Can you work these out from the model? Positions are in its coordinate system, mm. Face numbers are marked on the shaded views. A direction names the side the tool comes from. Coordinates: 2 decimals unless noted, no trailing zeros. Order: outer loops, then holes, each group sorted by start corner. A loop starts at its lowest first (then second) coordinate and runs counter-clockwise, first axis right, second up. Notation, with made-up numbers: M 69.25,-6.5 L 97.25,-6.5 A17 cw 97.25,17.5 Z; hole C 84,18.5 d11. An arc over 180 degrees is marked long. Answer as CSV lines item,"result". Start each with the question number.
1. I need wall thicknesses on line 1 along Y through (x, z) = (0, -16.3); line 2 along Y through (x, z) = (0, 0.5); line 3 along X through (y, z) = (-3, 27). Which ranges of each line are inside material? Lowest first, please. Write a range as from..to.
2. If we mould it in two halves opening along X, with no side actions, what happens to the marked faces 1, 2 and 3? For each: released by +X, released by -X, zero draft, split by the parting line, or undercut.
3. If we section it at A-A (z = 19.5): List the corners of the cut face in (x, y) for me, plus the area to 3 significant figures.
4. Will these pins go through, and if not, where does the flat tip stop? pin 1 (5 mm diameter, centred on x = -17.5, y = -9.5, fed in from -Z); pin 2 (8 mm diameter, centred on x = 4, z = -9.5, fed in from +Y); pin 3 (1 mm diameter, centred on x = -7.5, z = 3.5, fed in from +Y); pin 4 (20 mm diameter, centred on x = 0, y = 0, fed in from -Z).
5. If we section it at B-B (z = 27): List the corners of the cut face in (x, y) for me.
6. On a 3-axis mill with a long thin cutter (end or side, diameter ignored), from which of +Z, -Z, +X, -X, +Y, -Y can I reach the whole of each face in a straight line? I mean the marked faces 4 and 5. Say none if no direction works.
```python
from build123d import *


with BuildPart() as part:
    # Sketch1 → Revolve1 (revolve)
    with BuildSketch(Plane(origin=(0, 0, 0), x_dir=(1, 0, 0), z_dir=(0, 1, 0)), mode=Mode.PRIVATE) as revolve1_sk:
        with BuildLine():
            Line((-7.75, 0), (-7.75, 3.59874773))
            ThreePointArc((-7.75, 3.59874773), (-9.737150145, 8.834353772), (-9.25, 14.413154814))
            Line((-9.25, 14.413154814), (-9.25, 19.477254176))
            ThreePointArc((-9.25, 19.477254176), (-9.396446609, 19.830807566), (-9.75, 19.977254176))
            Line((-9.75, 19.977254176), (-10.624554433, 19.977254176))
            ThreePointArc((-10.624554433, 19.977254176), (-11.860926928, 19.63428676), (-12.743936524, 18.703406721))
            ThreePointArc((-12.743936524, 18.703406721), (-13.301894318, 17.444688456), (-13.4, 16.071348059))
            ThreePointArc((-13.4, 16.071348059), (-13.353676429, 16.020899185), (-13.300893142, 15.977254176))
            ThreePointArc((-13.300893142, 15.977254176), (-12.447206352, 14.854853584), (-12.371266932, 13.446735184))
            Line((-12.371266932, 13.446735184), (-14.64061089, 4.343335661))
            ThreePointArc((-14.64061089, 4.343335661), (-14.364146668, 2.750238564), (-13, 1.882197841))
            Line((-13, 1.882197841), (-13, 0))
            Line((-13, 0), (-27.863515915, -30.725250222))
            Line((-27.863515915, -30.725250222), (-7.75, -30.725250222))
            Line((-7.75, -30.725250222), (-7.75, 0))
        make_face()
    revolve(revolve1_sk.sketch.rotate(Axis((0, 0, 0), (0, 0, -1)), 180), axis=Axis((0, 0, 0), (0, 0, -1)))


solid = part.part
```
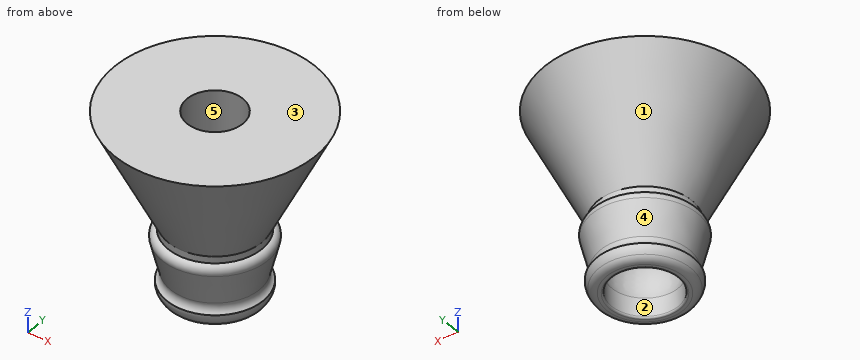
Solved:
1,line 1,"-13.42..-9.25, 9.25..13.42"
1,line 2,"-13.24..-7.75, 7.75..13.24"
1,line 3,"-25.89..-7.15, 7.15..25.89"
2,face 1,"split by the parting line"
2,face 2,"undercut"
2,face 3,"zero draft"
3,outline,"C 0,0 d44.87; hole C 0,0 d15.5"
3,area,"1,390 mm²"
4,pin 1,"z = 9.12"
4,pin 2,"y = 14.08"
4,pin 3,"y = 13.03"
4,pin 4,"z = -19.98"
5,outline,"C 0,0 d52.12; hole C 0,0 d15.5"
6,face 4,"none"
6,face 5,"+Z, -Z"
